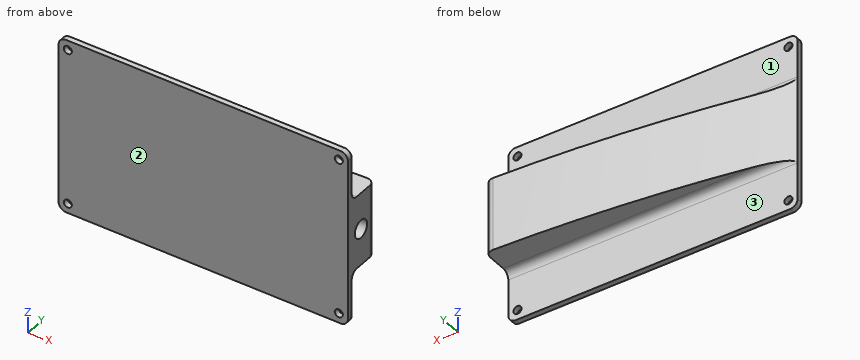
from build123d import *

# Parameters (mm, degrees)
SKETCH1_W                = 78.86
SKETCH1_H                = 48
BOSS_EXTRUDE1_DEPTH      = 1.5
CUT_EXTRUDE1_REACH       = 48.184
SKETCH2_R                = 1.1
FILLET1_R                = 2
BOSS_EXTRUDE2_DEPTH      = 10
BOSS_EXTRUDE2_DEPTH_BACK = 10
FILLET3_R                = 2
FILLET5_R                = 2
SKETCH4_R                = 2.45
CUT_EXTRUDE2_DEPTH       = 20


with BuildPart() as part:
    # Sketch1 → Boss-Extrude1 (new body)
    with BuildSketch(Plane(origin=(0, 0, 0), x_dir=(1, 0, 0), z_dir=(0, 1, 0))):
        Rectangle(SKETCH1_W, SKETCH1_H)
    extrude(amount=BOSS_EXTRUDE1_DEPTH)

    # Sketch2 → Cut-Extrude1 (cut, up to next)
    with BuildSketch(Plane(origin=(0, 1.5, 0), x_dir=(1, 0, 0), z_dir=(0, 1, 0)), mode=Mode.PRIVATE) as cut_extrude1_sk1:
        with Locations(Location((-36.93, 21.375, 0), (0, 0, 270))):
            Circle(SKETCH2_R)
    cut_extrude1_tool1 = extrude(cut_extrude1_sk1.sketch, amount=-CUT_EXTRUDE1_REACH, mode=Mode.PRIVATE) & part.part
    # Sketch2 → Cut-Extrude1 (cut, up to next)
    with BuildSketch(Plane(origin=(0, 1.5, 0), x_dir=(1, 0, 0), z_dir=(0, 1, 0)), mode=Mode.PRIVATE) as cut_extrude1_sk2:
        with Locations(Location((-36.93, -21.375, 0), (0, 0, 270))):
            Circle(SKETCH2_R)
    cut_extrude1_tool2 = extrude(cut_extrude1_sk2.sketch, amount=-CUT_EXTRUDE1_REACH, mode=Mode.PRIVATE) & part.part
    # Sketch2 → Cut-Extrude1 (cut, up to next)
    with BuildSketch(Plane(origin=(0, 1.5, 0), x_dir=(1, 0, 0), z_dir=(0, 1, 0)), mode=Mode.PRIVATE) as cut_extrude1_sk3:
        with Locations(Location((36.93, 21.375, 0), (0, 0, 270))):
            Circle(SKETCH2_R)
    cut_extrude1_tool3 = extrude(cut_extrude1_sk3.sketch, amount=-CUT_EXTRUDE1_REACH, mode=Mode.PRIVATE) & part.part
    # Sketch2 → Cut-Extrude1 (cut, up to next)
    with BuildSketch(Plane(origin=(0, 1.5, 0), x_dir=(1, 0, 0), z_dir=(0, 1, 0)), mode=Mode.PRIVATE) as cut_extrude1_sk4:
        with Locations(Location((36.93, -21.375, 0), (0, 0, 270))):
            Circle(SKETCH2_R)
    cut_extrude1_tool4 = extrude(cut_extrude1_sk4.sketch, amount=-CUT_EXTRUDE1_REACH, mode=Mode.PRIVATE) & part.part
    add(cut_extrude1_tool1.solids().sort_by_distance((-36.93, 1.5, -21.375))[0], mode=Mode.SUBTRACT)
    add(cut_extrude1_tool2.solids().sort_by_distance((-36.93, 1.5, 21.375))[0], mode=Mode.SUBTRACT)
    add(cut_extrude1_tool3.solids().sort_by_distance((36.93, 1.5, -21.375))[0], mode=Mode.SUBTRACT)
    add(cut_extrude1_tool4.solids().sort_by_distance((36.93, 1.5, 21.375))[0], mode=Mode.SUBTRACT)

    # Fillet1
    fillet1_edges = [part.edges().sort_by_distance(p)[0] for p in [
        (-39.43, 0.75, -24),
        (39.43, 0.75, -24),
        (39.43, 0.75, 24),
        (-39.43, 0.75, 24),
    ]]
    fillet(fillet1_edges, radius=FILLET1_R)

    # Sketch3 → Boss-Extrude2 (add, two sides: drawn at the far end of the back side and taken through both)
    with BuildSketch(Plane.XY.offset(-BOSS_EXTRUDE2_DEPTH_BACK)):
        with BuildLine():
            Line((39.43, 0.75), (39.43, 10.75))
            add(Edge.make_bspline(
                [(-39.43, 1.5), (-0.251175804, 9.517193524), (39.43, 10.75)],
                knots=[0, 0, 0, 1, 1, 1], degree=2))
            Line((-39.43, 1.5), (-39.43, 0.75))
            Line((-39.43, 0.75), (39.43, 0.75))
        make_face()
    extrude(amount=BOSS_EXTRUDE2_DEPTH + BOSS_EXTRUDE2_DEPTH_BACK)

    # Fillet3
    fillet3_edges = [part.edges().sort_by_distance(p)[0] for p in [
        (0, 1.5, 10),
        (0, 1.5, -10),
    ]]
    fillet(fillet3_edges, radius=FILLET3_R)

    # Fillet5
    fillet5_edges = [part.edges().sort_by_distance(p)[0] for p in [
        (39.43, 10.75, -5),
    ]]
    fillet(fillet5_edges, radius=FILLET5_R)

    # Sketch4 → Cut-Extrude2 (cut)
    with BuildSketch(Plane(origin=(39.43, 0, 0), x_dir=(0, 0, -1), z_dir=(1, 0, 0))):
        with Locations((0, 5.182287096)):
            Circle(SKETCH4_R)
    extrude(amount=-CUT_EXTRUDE2_DEPTH, mode=Mode.SUBTRACT)


solid = part.part
Design review of the part built by this model. Coordinates are the model's own, in mm. Face numbers are marked on the shaded views. A direction names the side the tool comes from. Coordinates: 2 decimals unless noted, no trailing zeros.
Item 1: For pin 1 Ø13 at (x, z) = (-9, 15) entering from +Y; pin 2 Ø2.5 at (x, z) = (36.93, -21.375) entering from +Y; pin 3 Ø5.5 at (x, y) = (0.5, 8) entering from -Z, all flat-tipped, find the tip position at first contact; note any pin that passes through.
Item 2: For line 1 (Y direction, x = 30, z = 0); line 2 (Y direction, x = 28.5, z = 12); line 3 (Z direction, x = -15, y = 4), list the stretches that pass through material, from the lowest coordinate up.
Item 3: For the marked faces 1, 2 and 3, list the 3-axis set-ups (+Z, -Z, +X, -X, +Y, -Y) from which the entire face can be reached by the end or side of a thin tool; tool diameter is ignored.
The answers:
1. pin 1: stops at y = 7.24
1. pin 2: stops at y = 1.5
1. pin 3: stops at z = -10
2. line 1: y = 0 to 2.73, 7.63 to 10.36
2. line 2: y = 0 to 1.5
2. line 3: z = -10 to 10
3. face 1: +Z, +X, -X, +Y
3. face 2: +Z, -Z, +X, -X, -Y
3. face 3: -Z, +X, -X, +Y
